Input: part model. Units: mm. Frame: model coordinates. A direction names the side the tool comes from. Coordinates: 2 decimals unless noted, no trailing zeros. Order: outer loops, then holes, each group sorted by start corner. A loop starts at its lowest first (then second) coordinate and runs counter-clockwise, first axis right, second up.
from build123d import *

# Parameters (mm, degrees)
F1_DEPTH = 330.2
F2_DEPTH = 3.175
F4_DEPTH = 53.975


with BuildPart() as f1:
    # F0 (on Front) → F1 (new body)
    with BuildSketch(Plane.XZ):
        Polygon((-134.881878, 63.5), (-134.881878, 0), (119.118122, 0), (117.848122, 3.175), (-131.706878, 3.175), (-131.706878, 60.325), (94.988122, 60.325), (93.718122, 63.5), align=None)
    extrude(amount=F1_DEPTH)

    # F0 (on Front) → F2 (join)
    with BuildSketch(Plane.XZ):
        Polygon((-131.706878, 3.175), (117.848122, 3.175), (94.988122, 60.325), (-131.706878, 60.325), align=None)
        Polygon((-134.881878, 63.5), (-134.881878, 0), (119.118122, 0), (117.848122, 3.175), (-131.706878, 3.175), (-131.706878, 60.325), (94.988122, 60.325), (93.718122, 63.5), align=None)
    extrude(amount=-F2_DEPTH)

    # F3 (on face) → F4 (join)
    with BuildSketch(Plane.XZ.offset(330.2)):
        Polygon((117.848122, 3.175), (94.988122, 60.325), (-131.706878, 60.325), (-131.706878, 3.175), align=None)
        Polygon((94.988122, 60.325), (93.718122, 63.5), (-134.881878, 63.5), (-134.881878, 0), (119.118122, 0), (117.848122, 3.175), (-131.706878, 3.175), (-131.706878, 60.325), align=None)
    extrude(amount=F4_DEPTH)


solid = f1.part
Item 1: Cut plane A-A on x = 54.5. Return loops of the section in (y, z) (3 decimals), then the cut area to 3 significant figures.
Response values:
outline: (-384.175, 0) - (3.175, 0) - (3.175, 63.5) - (-384.175, 63.5) - close; hole (-330.2, 3.175) - (0, 3.175) - (0, 60.325) - (-330.2, 60.325) - close
area: 5,730 mm2
Item 2: Access query for faces 1 (the face through (-10, -384.175, 32)), 2 (the face through (-20, -163, 60.325)). Directions: +Z, -Z, +X, -X, +Y, -Y. A direction counts if a zero-diameter tool reaches every point of the face in a straight line with its end or side. Return the directions, or none.
Response values:
face 1: +Z, -Z, +X, -X, -Y
face 2: +X
Item 3: Draft query along Z for faces 3 (the face through (-9, -330.2, 32)), 4 (the face through (-134.882, -188, 32)), 5 (the face through (-19, -188, 63.5)). Return one class per face: pulls with the +Z half, pulls with the -Z half, needs draft (parallel to the pull), parting line crosses it, or undercut.
Response values:
face 3: undercut
face 4: needs draft
face 5: pulls with the +Z half
Item 4: Cut plane B-B on y = -47. Return loops of the section in (x, z) (3 decimals), then the cut area to 3 significant figures.
Response values:
outline: (-134.882, 0) - (119.118, 0) - (117.848, 3.175) - (-131.707, 3.175) - (-131.707, 60.325) - (94.988, 60.325) - (93.718, 63.5) - (-134.882, 63.5) - close
area: 1,710 mm2
Item 5: Ray query, probe 1 along Y at (x, z) = (97, 13) (3 decimals); probe 2 along Z at (x, y) = (-17, -159) (3 decimals); probe 3 along X at (y, z) = (-223.5, 36.5). Return the intervals inside material, ascending.
Response values:
probe 1: y = -384.175 to -330.2, 0 to 3.175
probe 2: z = 0 to 3.175, 60.325 to 63.5
probe 3: x = -134.88 to -131.71
Item 6: Cut plane C-C on z = 38.5. Return loops of the section in (x, y) (3 decimals).
Response values:
outline: (-134.882, -384.175) - (103.718, -384.175) - (103.718, -330.2) - (-131.707, -330.2) - (-131.707, 0) - (103.718, 0) - (103.718, 3.175) - (-134.882, 3.175) - close
